from build123d import *

# Parameters (mm, degrees)
SKETCH1_W               = 25.4
SKETCH1_H               = 1397
SKETCH1_R               = 3.175
BOSS_EXTRUDE1_DEPTH     = 3.175
CUT_EXTRUDE1_DEPTH      = 699.622659685
CUT_EXTRUDE1_DEPTH_BACK = 699.622659685
SKETCH2_W               = 25.4
SKETCH2_H               = 1143


with BuildPart() as part:
    # Sketch1 → Boss-Extrude1 (new body)
    with BuildSketch(Plane(origin=(0, 0, 0), x_dir=(0, 0, -1), z_dir=(1, 0, 0))):
        Rectangle(SKETCH1_W, SKETCH1_H)
        with Locations((0, -685.8)):
            Circle(SKETCH1_R, mode=Mode.SUBTRACT)
        with Locations((0, -673.1)):
            Circle(SKETCH1_R, mode=Mode.SUBTRACT)
        with Locations((0, -660.4)):
            Circle(SKETCH1_R, mode=Mode.SUBTRACT)
        with Locations((0, -647.7)):
            Circle(SKETCH1_R, mode=Mode.SUBTRACT)
        with Locations((0, -635)):
            Circle(SKETCH1_R, mode=Mode.SUBTRACT)
        with Locations((0, -622.3)):
            Circle(SKETCH1_R, mode=Mode.SUBTRACT)
        with Locations((0, -609.6)):
            Circle(SKETCH1_R, mode=Mode.SUBTRACT)
        with Locations((0, -596.9)):
            Circle(SKETCH1_R, mode=Mode.SUBTRACT)
        with Locations((0, -584.2)):
            Circle(SKETCH1_R, mode=Mode.SUBTRACT)
        with Locations((0, -571.5)):
            Circle(SKETCH1_R, mode=Mode.SUBTRACT)
        with Locations((0, -558.8)):
            Circle(SKETCH1_R, mode=Mode.SUBTRACT)
        with Locations((0, -546.1)):
            Circle(SKETCH1_R, mode=Mode.SUBTRACT)
        with Locations((0, -533.4)):
            Circle(SKETCH1_R, mode=Mode.SUBTRACT)
        with Locations((0, -520.7)):
            Circle(SKETCH1_R, mode=Mode.SUBTRACT)
        with Locations((0, -508)):
            Circle(SKETCH1_R, mode=Mode.SUBTRACT)
        with Locations((0, -495.3)):
            Circle(SKETCH1_R, mode=Mode.SUBTRACT)
        with Locations((0, -482.6)):
            Circle(SKETCH1_R, mode=Mode.SUBTRACT)
        with Locations((0, -469.9)):
            Circle(SKETCH1_R, mode=Mode.SUBTRACT)
        with Locations((0, -457.2)):
            Circle(SKETCH1_R, mode=Mode.SUBTRACT)
        with Locations((0, -444.5)):
            Circle(SKETCH1_R, mode=Mode.SUBTRACT)
        with Locations((0, -431.8)):
            Circle(SKETCH1_R, mode=Mode.SUBTRACT)
        with Locations((0, -419.1)):
            Circle(SKETCH1_R, mode=Mode.SUBTRACT)
        with Locations((0, -406.4)):
            Circle(SKETCH1_R, mode=Mode.SUBTRACT)
        with Locations((0, -393.7)):
            Circle(SKETCH1_R, mode=Mode.SUBTRACT)
        with Locations((0, -381)):
            Circle(SKETCH1_R, mode=Mode.SUBTRACT)
        with Locations((0, -368.3)):
            Circle(SKETCH1_R, mode=Mode.SUBTRACT)
        with Locations((0, -355.6)):
            Circle(SKETCH1_R, mode=Mode.SUBTRACT)
        with Locations((0, -342.9)):
            Circle(SKETCH1_R, mode=Mode.SUBTRACT)
        with Locations((0, -330.2)):
            Circle(SKETCH1_R, mode=Mode.SUBTRACT)
        with Locations((0, -317.5)):
            Circle(SKETCH1_R, mode=Mode.SUBTRACT)
        with Locations((0, -304.8)):
            Circle(SKETCH1_R, mode=Mode.SUBTRACT)
        with Locations((0, -292.1)):
            Circle(SKETCH1_R, mode=Mode.SUBTRACT)
        with Locations((0, -279.4)):
            Circle(SKETCH1_R, mode=Mode.SUBTRACT)
        with Locations((0, -266.7)):
            Circle(SKETCH1_R, mode=Mode.SUBTRACT)
        with Locations((0, -254)):
            Circle(SKETCH1_R, mode=Mode.SUBTRACT)
        with Locations((0, -241.3)):
            Circle(SKETCH1_R, mode=Mode.SUBTRACT)
        with Locations((0, -228.6)):
            Circle(SKETCH1_R, mode=Mode.SUBTRACT)
        with Locations((0, -215.9)):
            Circle(SKETCH1_R, mode=Mode.SUBTRACT)
        with Locations((0, -203.2)):
            Circle(SKETCH1_R, mode=Mode.SUBTRACT)
        with Locations((0, -190.5)):
            Circle(SKETCH1_R, mode=Mode.SUBTRACT)
        with Locations((0, -177.8)):
            Circle(SKETCH1_R, mode=Mode.SUBTRACT)
        with Locations((0, -165.1)):
            Circle(SKETCH1_R, mode=Mode.SUBTRACT)
        with Locations((0, -152.4)):
            Circle(SKETCH1_R, mode=Mode.SUBTRACT)
        with Locations((0, -139.7)):
            Circle(SKETCH1_R, mode=Mode.SUBTRACT)
        with Locations((0, -127)):
            Circle(SKETCH1_R, mode=Mode.SUBTRACT)
        with Locations((0, -114.3)):
            Circle(SKETCH1_R, mode=Mode.SUBTRACT)
        with Locations((0, -101.6)):
            Circle(SKETCH1_R, mode=Mode.SUBTRACT)
        with Locations((0, -88.9)):
            Circle(SKETCH1_R, mode=Mode.SUBTRACT)
        with Locations((0, -76.2)):
            Circle(SKETCH1_R, mode=Mode.SUBTRACT)
        with Locations((0, -63.5)):
            Circle(SKETCH1_R, mode=Mode.SUBTRACT)
        with Locations((0, -50.8)):
            Circle(SKETCH1_R, mode=Mode.SUBTRACT)
        with Locations((0, -38.1)):
            Circle(SKETCH1_R, mode=Mode.SUBTRACT)
        with Locations((0, -25.4)):
            Circle(SKETCH1_R, mode=Mode.SUBTRACT)
        with Locations((0, -12.7)):
            Circle(SKETCH1_R, mode=Mode.SUBTRACT)
        Circle(SKETCH1_R, mode=Mode.SUBTRACT)
        with Locations((0, 12.7)):
            Circle(SKETCH1_R, mode=Mode.SUBTRACT)
        with Locations((0, 25.4)):
            Circle(SKETCH1_R, mode=Mode.SUBTRACT)
        with Locations((0, 38.1)):
            Circle(SKETCH1_R, mode=Mode.SUBTRACT)
        with Locations((0, 50.8)):
            Circle(SKETCH1_R, mode=Mode.SUBTRACT)
        with Locations((0, 63.5)):
            Circle(SKETCH1_R, mode=Mode.SUBTRACT)
        with Locations((0, 76.2)):
            Circle(SKETCH1_R, mode=Mode.SUBTRACT)
        with Locations((0, 88.9)):
            Circle(SKETCH1_R, mode=Mode.SUBTRACT)
        with Locations((0, 101.6)):
            Circle(SKETCH1_R, mode=Mode.SUBTRACT)
        with Locations((0, 114.3)):
            Circle(SKETCH1_R, mode=Mode.SUBTRACT)
        with Locations((0, 127)):
            Circle(SKETCH1_R, mode=Mode.SUBTRACT)
        with Locations((0, 139.7)):
            Circle(SKETCH1_R, mode=Mode.SUBTRACT)
        with Locations((0, 152.4)):
            Circle(SKETCH1_R, mode=Mode.SUBTRACT)
        with Locations((0, 165.1)):
            Circle(SKETCH1_R, mode=Mode.SUBTRACT)
        with Locations((0, 177.8)):
            Circle(SKETCH1_R, mode=Mode.SUBTRACT)
        with Locations((0, 190.5)):
            Circle(SKETCH1_R, mode=Mode.SUBTRACT)
        with Locations((0, 203.2)):
            Circle(SKETCH1_R, mode=Mode.SUBTRACT)
        with Locations((0, 215.9)):
            Circle(SKETCH1_R, mode=Mode.SUBTRACT)
        with Locations((0, 228.6)):
            Circle(SKETCH1_R, mode=Mode.SUBTRACT)
        with Locations((0, 241.3)):
            Circle(SKETCH1_R, mode=Mode.SUBTRACT)
        with Locations((0, 254)):
            Circle(SKETCH1_R, mode=Mode.SUBTRACT)
        with Locations((0, 266.7)):
            Circle(SKETCH1_R, mode=Mode.SUBTRACT)
        with Locations((0, 279.4)):
            Circle(SKETCH1_R, mode=Mode.SUBTRACT)
        with Locations((0, 292.1)):
            Circle(SKETCH1_R, mode=Mode.SUBTRACT)
        with Locations((0, 304.8)):
            Circle(SKETCH1_R, mode=Mode.SUBTRACT)
        with Locations((0, 317.5)):
            Circle(SKETCH1_R, mode=Mode.SUBTRACT)
        with Locations((0, 330.2)):
            Circle(SKETCH1_R, mode=Mode.SUBTRACT)
        with Locations((0, 342.9)):
            Circle(SKETCH1_R, mode=Mode.SUBTRACT)
        with Locations((0, 355.6)):
            Circle(SKETCH1_R, mode=Mode.SUBTRACT)
        with Locations((0, 368.3)):
            Circle(SKETCH1_R, mode=Mode.SUBTRACT)
        with Locations((0, 381)):
            Circle(SKETCH1_R, mode=Mode.SUBTRACT)
        with Locations((0, 393.7)):
            Circle(SKETCH1_R, mode=Mode.SUBTRACT)
        with Locations((0, 406.4)):
            Circle(SKETCH1_R, mode=Mode.SUBTRACT)
        with Locations((0, 419.1)):
            Circle(SKETCH1_R, mode=Mode.SUBTRACT)
        with Locations((0, 431.8)):
            Circle(SKETCH1_R, mode=Mode.SUBTRACT)
        with Locations((0, 444.5)):
            Circle(SKETCH1_R, mode=Mode.SUBTRACT)
        with Locations((0, 457.2)):
            Circle(SKETCH1_R, mode=Mode.SUBTRACT)
        with Locations((0, 469.9)):
            Circle(SKETCH1_R, mode=Mode.SUBTRACT)
        with Locations((0, 482.6)):
            Circle(SKETCH1_R, mode=Mode.SUBTRACT)
        with Locations((0, 495.3)):
            Circle(SKETCH1_R, mode=Mode.SUBTRACT)
        with Locations((0, 508)):
            Circle(SKETCH1_R, mode=Mode.SUBTRACT)
        with Locations((0, 520.7)):
            Circle(SKETCH1_R, mode=Mode.SUBTRACT)
        with Locations((0, 533.4)):
            Circle(SKETCH1_R, mode=Mode.SUBTRACT)
        with Locations((0, 546.1)):
            Circle(SKETCH1_R, mode=Mode.SUBTRACT)
        with Locations((0, 558.8)):
            Circle(SKETCH1_R, mode=Mode.SUBTRACT)
        with Locations((0, 571.5)):
            Circle(SKETCH1_R, mode=Mode.SUBTRACT)
        with Locations((0, 584.2)):
            Circle(SKETCH1_R, mode=Mode.SUBTRACT)
        with Locations((0, 596.9)):
            Circle(SKETCH1_R, mode=Mode.SUBTRACT)
        with Locations((0, 609.6)):
            Circle(SKETCH1_R, mode=Mode.SUBTRACT)
        with Locations((0, 622.3)):
            Circle(SKETCH1_R, mode=Mode.SUBTRACT)
        with Locations((0, 635)):
            Circle(SKETCH1_R, mode=Mode.SUBTRACT)
        with Locations((0, 647.7)):
            Circle(SKETCH1_R, mode=Mode.SUBTRACT)
        with Locations((0, 660.4)):
            Circle(SKETCH1_R, mode=Mode.SUBTRACT)
        with Locations((0, 673.1)):
            Circle(SKETCH1_R, mode=Mode.SUBTRACT)
        with Locations((0, 685.8)):
            Circle(SKETCH1_R, mode=Mode.SUBTRACT)
    extrude(amount=BOSS_EXTRUDE1_DEPTH)

    # Sketch2 → Cut-Extrude1 (cut, two sides: drawn at the far end of the back side and taken through both)
    with BuildSketch(Plane(origin=(3.175, 0, 0), x_dir=(0, 0, -1), z_dir=(1, 0, 0)).offset(-CUT_EXTRUDE1_DEPTH_BACK)):
        with Locations((0, 127)):
            Rectangle(SKETCH2_W, SKETCH2_H)
    extrude(amount=CUT_EXTRUDE1_DEPTH + CUT_EXTRUDE1_DEPTH_BACK, mode=Mode.SUBTRACT)


solid = part.part
CAD build for the part. Positions are in the model's coordinates, mm. Round coordinates to 2 decimals unless told otherwise and drop trailing zeros. Loops run counter-clockwise (first coordinate to the right, second up) from the corner with the lowest first, then second, coordinate; pieces in that order, holes last.
(1) Drop a flat-ended pin along its axis: pin 1 (10 mm diameter, centred on y = -508, z = 0, fed in from +X) (3 decimals). Give the stop position or say it passes through.
(2) Cut at A-A (y = -469.9). Give the cut face in (x, z) (3 decimals), plus the area to 3 significant figures.
(3) Two-plate mould, pull along Z, no slides. Class faces 1 (the cylindrical face through (1.57, -669.95, 0.41)), 2 (the flat face through (3.175, -570, 3)): +Z half, -Z half, draft (parallel to the pull), parting line (faces both ways), or undercut.
(4) Wall check: line 1 along Z through (x, y) = (2.05, -482.6) (3 decimals); line 2 along Z through (x, y) = (0.75, -548). Give the ranges that are in metal, low to high.
(5) Cut at B-B (x = 1.9). State how many separate pieces and enclosed holes the cut face has, plus the area to 3 significant figures.
Findings below:
1. pin 1: stops at x = 3.175
2. outline: (0, -12.7) - (3.175, -12.7) - (3.175, -3.175) - (0, -3.175) - close; (0, 3.175) - (3.175, 3.175) - (3.175, 12.7) - (0, 12.7) - close
2. area: 60.5 mm2
3. face 1: undercut
3. face 2: draft
4. line 1: z = -12.7 to -3.175, 3.175 to 12.7
4. line 2: z = -12.7 to -2.54, 2.54 to 12.7
5. separate pieces: 1
5. enclosed holes: 19
5. area: 5,830 mm2
